```python
from build123d import *

# Parameters (mm, degrees)
BOSS_EXTRUDE1_DEPTH                                 = 500
CBORE_FOR_M6_HEX_SOCKET_HEAD_CAP_SCREW1_D           = 7
CBORE_FOR_M6_HEX_SOCKET_HEAD_CAP_SCREW1_CBORE_D     = 11
CBORE_FOR_M6_HEX_SOCKET_HEAD_CAP_SCREW1_CBORE_DEPTH = 9
LPATTERN1_COUNT                                     = 9
LPATTERN1_PITCH                                     = 60


with BuildPart() as part:
    # Sketch1 → Boss-Extrude1 (new body)
    with BuildSketch(Plane.XY):
        with BuildLine():
            Line((-8.192893219, -12.452822372), (-11.5, -15.759929153))
            Line((-11.5, -15.759929153), (-11.5, -17))
            Line((-11.5, -17), (-10.5, -18))
            Line((-10.5, -18), (10.5, -18))
            Line((10.5, -18), (11.5, -17))
            Line((11.5, -17), (11.5, -15.759929153))
            Line((11.5, -15.759929153), (8.192893219, -12.452822372))
            ThreePointArc((8.192893219, -12.452822372), (7.976120468, -12.128399023), (7.9, -11.745715591))
            Line((7.9, -11.745715591), (7.9, -8.934076562))
            ThreePointArc((7.9, -8.934076562), (7.976120468, -8.55139313), (8.192893219, -8.226969781))
            Line((8.192893219, -8.226969781), (8.93515621, -7.48470679))
            ThreePointArc((8.93515621, -7.48470679), (9.020912002, -7.369915712), (9.070589884, -7.235516473))
            ThreePointArc((9.070589884, -7.235516473), (9.728797536, -6.024451536), (10.939862473, -5.366243884))
            ThreePointArc((10.939862473, -5.366243884), (11.074261712, -5.316566002), (11.18905279, -5.23081021))
            Line((11.18905279, -5.23081021), (11.353553391, -5.066309609))
            ThreePointArc((11.353553391, -5.066309609), (11.461939766, -4.904097935), (11.5, -4.712756219))
            Line((11.5, -4.712756219), (11.5, -3.298408781))
            ThreePointArc((11.5, -3.298408781), (11.461939766, -3.107067065), (11.353553391, -2.944855391))
            Line((11.353553391, -2.944855391), (11.175123458, -2.766425458))
            ThreePointArc((11.175123458, -2.766425458), (11.061399997, -2.681251593), (10.928310161, -2.631505152))
            ThreePointArc((10.928310161, -2.631505152), (9.728797536, -1.975792464), (9.073084848, -0.776279839))
            ThreePointArc((9.073084848, -0.776279839), (9.023338407, -0.643190003), (8.938164542, -0.529466542))
            Line((8.938164542, -0.529466542), (8.408698, 0))
            Line((8.408698, 0), (-8.408698, 0))
            Line((-8.408698, 0), (-8.938164542, -0.529466542))
            ThreePointArc((-8.938164542, -0.529466542), (-9.023338407, -0.643190003), (-9.073084848, -0.776279839))
            ThreePointArc((-9.073084848, -0.776279839), (-9.728797536, -1.975792464), (-10.928310161, -2.631505152))
            ThreePointArc((-10.928310161, -2.631505152), (-11.061399997, -2.681251593), (-11.175123458, -2.766425458))
            Line((-11.175123458, -2.766425458), (-11.353553391, -2.944855391))
            ThreePointArc((-11.353553391, -2.944855391), (-11.461939766, -3.107067065), (-11.5, -3.298408781))
            Line((-11.5, -3.298408781), (-11.5, -4.712756219))
            ThreePointArc((-11.5, -4.712756219), (-11.461939766, -4.904097935), (-11.353553391, -5.066309609))
            Line((-11.353553391, -5.066309609), (-11.18905279, -5.23081021))
            ThreePointArc((-11.18905279, -5.23081021), (-11.074261712, -5.316566002), (-10.939862473, -5.366243884))
            ThreePointArc((-10.939862473, -5.366243884), (-9.728797536, -6.024451536), (-9.070589884, -7.235516473))
            ThreePointArc((-9.070589884, -7.235516473), (-9.020912002, -7.369915712), (-8.93515621, -7.48470679))
            Line((-8.93515621, -7.48470679), (-8.192893219, -8.226969781))
            ThreePointArc((-8.192893219, -8.226969781), (-7.976120468, -8.55139313), (-7.9, -8.934076562))
            Line((-7.9, -8.934076562), (-7.9, -11.745715591))
            ThreePointArc((-7.9, -11.745715591), (-7.976120468, -12.128399023), (-8.192893219, -12.452822372))
        make_face()
    extrude(amount=BOSS_EXTRUDE1_DEPTH)

    # CBORE for M6 Hex Socket Head Cap Screw1 (through all)
    with Locations(Plane(origin=(0, 0, 10), x_dir=(0, 0, 1), z_dir=(0, 1, 0))):
        with Locations((0, 0)):
            cbore_for_m6_hex_socket_head_cap_screw1 = CounterBoreHole(CBORE_FOR_M6_HEX_SOCKET_HEAD_CAP_SCREW1_D / 2, CBORE_FOR_M6_HEX_SOCKET_HEAD_CAP_SCREW1_CBORE_D / 2, CBORE_FOR_M6_HEX_SOCKET_HEAD_CAP_SCREW1_CBORE_DEPTH)

    # LPattern1: CBORE for M6 Hex Socket Head Cap Screw1 ×9
    with Locations(*[(0, 0, i * LPATTERN1_PITCH) for i in range(1, LPATTERN1_COUNT)]):
        add(cbore_for_m6_hex_socket_head_cap_screw1, mode=Mode.SUBTRACT)


solid = part.part
```
Build history of the part. All positions in model axes, mm. A direction names the side the tool comes from. Give positions to 0.01 mm unless a question says otherwise; leave off trailing zeros. One line per question, with ' | ' between items. Start each with the question number.
1) Pin check, flat tips, straight feed: pin 1 (6 mm diameter, centred on y = -9.5, z = 355.5, fed in from +X); pin 2 (3.5 mm diameter, centred on x = 0.5, z = 492.5, fed in from +Y); pin 3 (1 mm diameter, centred on y = -6.5, z = 299.5, fed in from -X). Stop position of each tip, or through.
2) Probe L1, parallel to X at y = -16, z = 70; L2, parallel to X at y = -5, z = 317.5; L3, parallel to Y at x = -10.25, z = 267.5. List the from-to ranges inside material, lowest first.
3) Two-plate mould, pull along X, no slides. Class faces 3 (the cylindrical face through (1.652, -4.437, 435.246)), 4 (the flat face through (-4, -9, 370)), 5 (the flat face through (0, -9, 500)): released by +X, released by -X, zero draft, split by the parting line, or undercut.
4) Cut at A-A (x = 0). Count the separate pieces of the cut face and the enclosed holes in it, plus the area to 3 significant figures.
5) 3-axis set-ups, long thin cutter, end or side, ignore diameter. For faces 1 (the flat face through (0, -9, 314)), 2 (the flat face through (0, -9, 0)): which of +Z, -Z, +X, -X, +Y, -Y reach the whole face in a straight line?
Return value:
1) pin 1: x = 9.36 | pin 2: y = -9 | pin 3: x = -9.75
2) L1: -11.5 to -3.5, 3.5 to 11.5 | L2: -11.41 to 11.41 | L3: -18 to -14.51, -5.63 to -2.37
3) face 3: undercut | face 4: undercut | face 5: zero draft
4) separate pieces: 10 | enclosed holes: 0 | area: 7,540 mm^2
5) face 1: +Y | face 2: -Z, +X, -X, +Y, -Y
